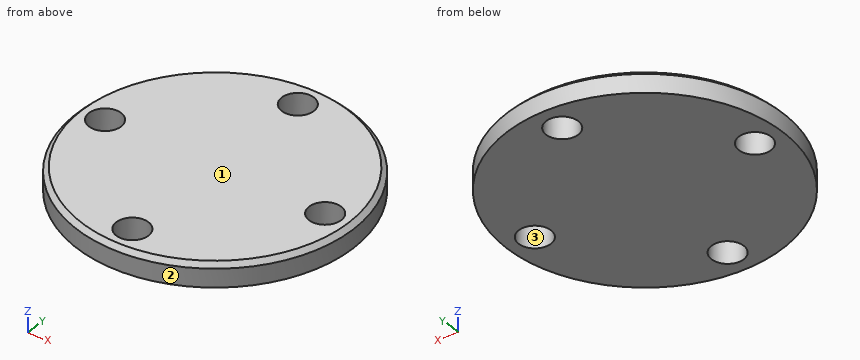
```python
from build123d import *

# Parameters (mm, degrees)
F0_R     = 15
F0_R_2   = 1.75
F0_R_3   = 6.5
F1_DEPTH = 2.5
F2_SIZE  = 0.5


with BuildPart() as f1:
    # F0 (on Top) → F1 (new body)
    with BuildSketch(Plane.XY):
        Circle(F0_R)
        with Locations((0, -12)):
            Circle(F0_R_2, mode=Mode.SUBTRACT)
        with Locations((-12, 0)):
            Circle(F0_R_2, mode=Mode.SUBTRACT)
        Circle(F0_R_3, mode=Mode.SUBTRACT)
        with Locations((12, 0)):
            Circle(F0_R_2, mode=Mode.SUBTRACT)
        with Locations((0, 12)):
            Circle(F0_R_2, mode=Mode.SUBTRACT)
        Circle(F0_R_3)
    extrude(amount=F1_DEPTH)

    # F2
    f2_edges = [f1.edges().sort_by_distance(p)[0] for p in [
        (-15, 0, 2.5),
    ]]
    chamfer(f2_edges, length=F2_SIZE)


solid = f1.part
```
Work out the finished part from the listing and answer in its coordinate system (mm). Face numbers are marked on the shaded views. Give positions to 0.01 mm unless a question says otherwise; leave off trailing zeros. Write each loop counter-clockwise with the first axis right and the second up, starting at its lowest first coordinate (ties: lowest second). Pieces come first, ordered by that corner, then holes.
(1) The part is cut by section A-A on x = 0. Write down the section's boundary in (y, z).
Final values:
outline: (-15, 0) - (-13.75, 0) - (-13.75, 2.5) - (-14.5, 2.5) - (-15, 2) - close; (-10.25, 0) - (10.25, 0) - (10.25, 2.5) - (-10.25, 2.5) - close; (13.75, 0) - (15, 0) - (15, 2) - (14.5, 2.5) - (13.75, 2.5) - close
(2) Straight lines are drawn through the part: line 1 (Y direction, x = 0, z = 0.65); line 2 (Y direction, x = 0, z = 2.35); line 3 (Y direction, x = -12, z = 1.9). For each, find the intervals that lie inside material, in ascending order.
Final values:
line 1: y = -15 to -13.75, -10.25 to 10.25, 13.75 to 15
line 2: y = -14.65 to -13.75, -10.25 to 10.25, 13.75 to 14.65
line 3: y = -9 to -1.75, 1.75 to 9
(3) The part is cut by section C-C on z = 1.1. Write down the section's boundary in (x, y).
Final values:
outline: circle Ø30 at (0, 0); hole circle Ø3.5 at (-12, 0); hole circle Ø3.5 at (0, -12); hole circle Ø3.5 at (0, 12); hole circle Ø3.5 at (12, 0)
(4) The mould has two halves that part along X. Classify the marked faces 1, 2 and 3: pulls with the +X half, pulls with the -X half, needs draft (parallel to the pull), parting line crosses it, or undercut.
Final values:
face 1: needs draft
face 2: parting line crosses it
face 3: undercut
(5) Flat-ended cylindrical pins translate along their axes: pin 1 Ø3 at (x, y) = (12, 0) entering from +Z; pin 2 Ø1 at (y, z) = (11, 2) entering from +X. Find the tip coordinate at first contact, or state that the pin passes through.
Final values:
pin 1: passes through
pin 2: stops at x = 10.71
